from build123d import *

# Parameters (mm, degrees)
SKETCH15_R          = 17
SKETCH15_R_2        = 16
BOSS_EXTRUDE1_DEPTH = 5
BOSS_EXTRUDE2_DEPTH = 1.5
CIRPATTERN1_COUNT   = 12


with BuildPart() as part:
    # Sketch15 → Boss-Extrude1 (new body)
    with BuildSketch(Plane.XY):
        Circle(SKETCH15_R)
        Circle(SKETCH15_R_2, mode=Mode.SUBTRACT)
    extrude(amount=BOSS_EXTRUDE1_DEPTH)

    # Sketch16 → Boss-Extrude2 (add, symmetric)
    with BuildSketch(Plane(origin=(0, 0, 2.5), x_dir=(-1, 0, 0), z_dir=(0, 0, -1))):
        with BuildLine():
            Line((2.5, 14.803480629), (2.5, 15.803480629))
            ThreePointArc((2.5, 15.803480629), (0, 16), (-2.5, 15.803480629))
            Line((-2.5, 15.803480629), (-2.5, 14.803480629))
            Line((-2.5, 14.803480629), (2.5, 14.803480629))
        make_face()
    boss_extrude2 = extrude(amount=BOSS_EXTRUDE2_DEPTH, both=True)

    # CirPattern1: Boss-Extrude2 ×12 about axis
    cirpattern1_axis = Axis((0, 0, 0), (0, 0, 1))
    for i in range(1, CIRPATTERN1_COUNT):
        add(boss_extrude2.rotate(cirpattern1_axis, i * 360 / CIRPATTERN1_COUNT))


solid = part.part
Build history of the part. All positions in model axes, mm. A direction names the side the tool comes from. Round coordinates to 2 decimals unless told otherwise and drop trailing zeros. Write each loop counter-clockwise with the first axis right and the second up, starting at its lowest first coordinate (ties: lowest second). Pieces come first, ordered by that corner, then holes. Notation, with made-up numbers: (-17, -2.75) -> (19, -2.75) arc R9 cw to (19, 13.25) -> close; hole circle Ø11 at (-36.5, -35.75). An arc over 180 degrees is marked (long way). Write item = value, one per line.
(1) Band-saw the part on C-C (x = 3.5). Give the cut face in (y, z).
Answer:
outline = (-16.64, 0) -> (-15.61, 0) -> (-15.61, 5) -> (-16.64, 5) -> close; (15.61, 0) -> (16.64, 0) -> (16.64, 5) -> (15.61, 5) -> close
(2) Band-saw the part on D-D (y = 11). Give the cut face in (x, z).
Answer:
outline = (-12.96, 0) -> (-11.62, 0) -> (-11.62, 5) -> (-12.96, 5) -> close; (11.62, 0) -> (12.96, 0) -> (12.96, 5) -> (11.62, 5) -> close
(3) Flat gauge pins, fed straight in: pin 1 (1.5 mm diameter, centred on y = -12.5, z = 2.5, fed in from -X); pin 2 (0.5 mm diameter, centred on y = 15.5, z = 2.5, fed in from -X); pin 3 (1 mm diameter, centred on x = 7.5, y = -12.5, fed in from -Z). Where does each tip first touch, or does it go through?
Answer:
pin_1 = -12.29
pin_2 = -7.51
pin_3 = 1
(4) Two-plate mould, pull along X, no slides. Class faces 4 (the face through (15, 2.5, 2)), 5 (the face through (9.139, 14.334, 2.465)), 6 (the face through (13, -10, 5)): pulls with the +X half, pulls with the -X half, needs draft (parallel to the pull), parting line crosses it, or undercut.
Answer:
face_4 = undercut
face_5 = parting line crosses it
face_6 = needs draft
(5) Tool access for faces 1 (the face through (13, 8, 4)), 2 (the face through (9.82, 12.01, 2.48)), 3 (the face through (-13, -8, 1)): list every direction of +Z, -Z, +X, -X, +Y, -Y with a clear straight run to the whole face (end or side of a thin tool).
Answer:
face_1 = +Z
face_2 = +Z, -Z
face_3 = -Z
(6) Probe L1, parallel to Y at x = 0, z = 2.7; L2, parallel to X at y = -0.5, z = 3.8; L3, parallel to X at y = -5.5, z = 2.4. List the from-to ranges inside material, lowest first.
Answer:
L1 = -17 to -14.8, 14.8 to 17
L2 = -16.99 to -14.8, 14.8 to 16.99
L3 = -16.09 to -15.02, -14.53 to -13.92, 13.92 to 14.53, 15.02 to 16.09
(7) Band-saw the part on A-A (y = 0). Give the cut face in (x, z).
Answer:
outline = (-17, 0) -> (-16, 0) -> (-16, 1) -> (-14.8, 1) -> (-14.8, 4) -> (-16, 4) -> (-16, 5) -> (-17, 5) -> close; (14.8, 1) -> (16, 1) -> (16, 0) -> (17, 0) -> (17, 5) -> (16, 5) -> (16, 4) -> (14.8, 4) -> close
